from build123d import *

# Parameters (mm, degrees)
SKETCH_1_R          = 2.5
EXTRUDE_1_DEPTH     = 80
SKETCH_2_W          = 20
SKETCH_2_H          = 15
CUT_EXTRUDE_1_DEPTH = 80


with BuildPart() as part:
    # 草图1 → 凸台-拉伸1 (new body)
    with BuildSketch(Plane.XY):
        with BuildLine():
            Line((-5, 10), (5, 10))
            Line((5, 10), (5, 0))
            ThreePointArc((5, 0), (0, -5), (-5, 0))
            Line((-5, 0), (-5, 10))
        make_face()
        Circle(SKETCH_1_R, mode=Mode.SUBTRACT)
    extrude(amount=EXTRUDE_1_DEPTH)

    # 草图2 → 切除-拉伸1 (cut)
    with BuildSketch(Plane(origin=(5, 0, 0), x_dir=(0, 0, -1), z_dir=(1, 0, 0))):
        with Locations((-15, -2.5)):
            Rectangle(SKETCH_2_W, SKETCH_2_H)
        with Locations((-65, -2.5)):
            Rectangle(SKETCH_2_W, SKETCH_2_H)
    extrude(amount=-CUT_EXTRUDE_1_DEPTH, mode=Mode.SUBTRACT)


solid = part.part
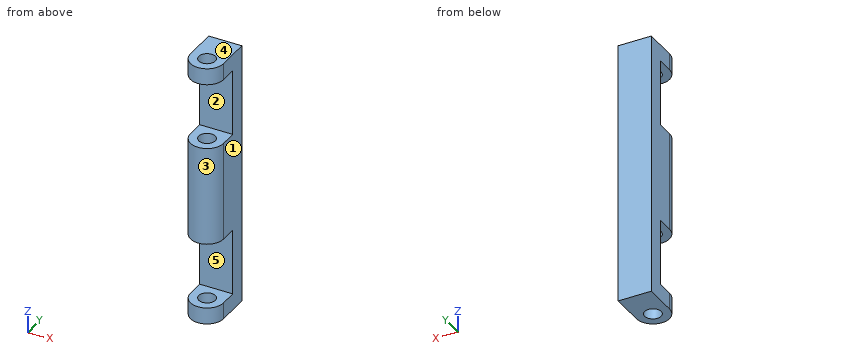
Model file for the job. Use its own axes, mm. Face numbers are marked on the shaded views. A direction names the side the tool comes from. Round coordinates to 2 decimals unless told otherwise and drop trailing zeros. Loops run counter-clockwise (first coordinate to the right, second up) from the corner with the lowest first, then second, coordinate; pieces in that order, holes last.
1. Tool access for the marked faces 1 and 2: list every direction of +Z, -Z, +X, -X, +Y, -Y with a clear straight run to the whole face (end or side of a thin tool).
Check values:
face 1: +Z, -Z, +X, +Y, -Y
face 2: +X, -X, -Y
2. Band-saw the part on B-B, the plane x = 0. List the corners of the cut face in (y, z), and give its area (3 significant figures).
Check values:
outline: (-5, 0) - (-2.5, 0) - (-2.5, 5) - (-5, 5) - close; (-5, 25) - (-2.5, 25) - (-2.5, 55) - (-5, 55) - close; (-5, 75) - (-2.5, 75) - (-2.5, 80) - (-5, 80) - close; (2.5, 0) - (10, 0) - (10, 80) - (2.5, 80) - (2.5, 75) - (5, 75) - (5, 55) - (2.5, 55) - (2.5, 25) - (5, 25) - (5, 5) - (2.5, 5) - close
area: 600 mm2
3. Band-saw the part on D-D, the plane x = -4. List the corners of the cut face in (y, z), and give its area (3 significant figures).
Check values:
outline: (-3, 0) - (10, 0) - (10, 80) - (-3, 80) - (-3, 75) - (5, 75) - (5, 55) - (-3, 55) - (-3, 25) - (5, 25) - (5, 5) - (-3, 5) - close
area: 720 mm2
4. Mould opens along Z. For the marked faces 3, 4 and 5 say: +Z half, -Z half, draft (parallel to the pull), parting line (faces both ways), or undercut.
Check values:
face 3: draft
face 4: +Z half
face 5: undercut
5. Band-saw the part on C-C, the plane z = 47. List the corners of the cut face in (x, y), and give its area (3 significant figures).
Check values:
outline: (-5, 0) arc R5 ccw to (5, 0) - (5, 10) - (-5, 10) - close; hole circle Ø5 at (0, 0)
area: 120 mm2
6. Wall check: probe 1 along Z at (x, y) = (1.5, -2.25); probe 2 along Y at (x, z) = (0, 47.25); probe 3 along X at (y, z) = (0, 76.6). Give the ranges that are in metal, low to high.
Check values:
probe 1: z = 0 to 5, 25 to 55, 75 to 80
probe 2: y = -5 to -2.5, 2.5 to 10
probe 3: x = -5 to -2.5, 2.5 to 5
7. Drop a flat-ended pin along its axis: P1, Ø3, axis at x = 0, z = 64, coming from the -Y side. Give the stop position or say it passes through.
Check values:
P1: stops at y = 5
8. Band-saw the part on A-A, the plane y = 3.5. List the corners of the cut face in (x, z), and give its area (3 significant figures).
Check values:
outline: (-5, 0) - (5, 0) - (5, 5) - (-5, 5) - close; (-5, 25) - (5, 25) - (5, 55) - (-5, 55) - close; (-5, 75) - (5, 75) - (5, 80) - (-5, 80) - close
area: 400 mm2
